Autodesk Inventor part; units mm, degrees
ref_plane "YZ Plane" through (0, 0, 0) normal (1, 0, 0) x (0, 1, 0)
ref_plane "XZ Plane" through (0, 0, 0) normal (0, 1, 0) x (-1, 0, 0)
ref_plane "XY Plane" through (0, 0, 0) normal (0, 0, 1) x (1, 0, 0)
sketch "Sketch1" plane through (0, 0, 0) normal (0, 1, 0) x (-1, 0, 0)
  line L0 (0, 0) -> (80, 0)
  line L1 (80, 0) -> (80, -40)
  line L2 (80, -40) -> (0, -40)
  line L3 (0, -40) -> (0, 0)
  line L4 (0, 0) -> (10, 0)
  line L5 (10, 0) -> (10, -10)
  line L6 (10, -10) -> (10, -30)
  circle A0 centre (10, -10) radius 3
  circle A1 centre (10, -30) radius 3
  line L7 (80, 0) -> (60, 0)
  line L8 (60, 0) -> (60, 30)
  line L9 (60, 30) -> (80, 30)
  line L10 (80, 30) -> (80, 0)
  dimension "d0" = 80
  dimension "d1" = 40
  dimension "d2" = 10
  dimension "d3" = 10
  dimension "d4" = 20
  dimension "d5" = 6
  dimension "d6" = 6
  dimension "d28" = 20
  dimension "d29" = 30
extrude "Extrusion1" add sketch "Sketch1" along normal blind 6
fillet "Fillet5" radius 5 6 edges at (-60, 3, 0) (-60, 3, 30) (-80, 3, 30) (0, 3, 0) (0, 3, -40) (-80, 3, -40)
fillet "Fillet6" radius 3 24 edges at (-1.4645, 6, -1.4645) (0, 6, -20) (-1.4645, 6, -38.5355) (-40, 6, -40) (-78.5355, 6, -38.5355) (-80, 6, -5) (-78.5355, 6, 28.5355) (-70, 6, 30) (-61.4645, 6, 28.5355) (-60, 6, 15) (-58.5355, 6, 1.4645) (-30, 6, 0) (-1.4645, 0, -1.4645) (0, 0, -20) (-1.4645, 0, -38.5355) (-40, 0, -40) (-78.5355, 0, -38.5355) (-80, 0, -5) (-78.5355, 0, 28.5355) (-70, 0, 30) (-61.4645, 0, 28.5355) (-60, 0, 15) (-58.5355, 0, 1.4645) (-30, 0, 0)
properties part number "CableHook"
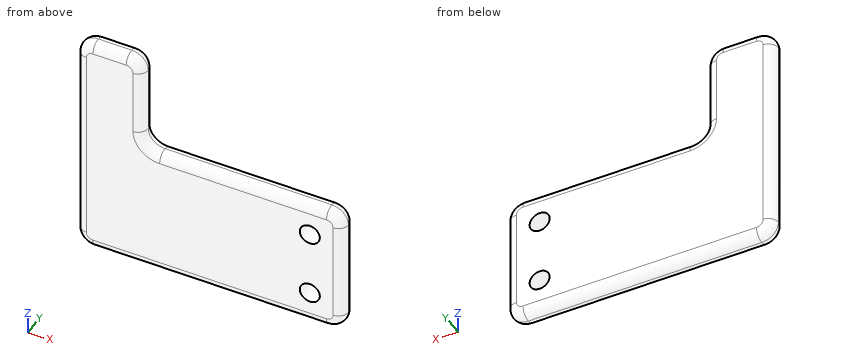
The listing builds one solid part. Answer for the finished solid, in the listing's coordinates (mm). Coordinates: 2 decimals unless noted, no trailing zeros.
Q1. Given P1, Ø9.5, axis at x = -10, z = -10, coming from the +Y side; P2, Ø1, axis at x = -22.5, y = 1.5, coming from the +Z side; P3, Ø2, axis at x = -27, y = 2, coming from the +Z side; P4, Ø1, axis at y = 2, z = 22.5, coming from the +X side, each flat-ended and moving along its own axis, determine where each tip first touches the part or whether it passes through.
Q2. A cutting plane is placed at B-B, the plane x = -10. State how many separate pieces and enclosed holes the cut face has, and give its area (3 significant figures).
Q3. Consider line 1 (Z direction, x = -10, y = 3.05); line 2 (X direction, y = 2.8, z = -10); line 3 (X direction, y = 3.85, z = -30). Determine where each line is inside the solid, lowest interval first.
Answers follow:
1. P1: stops at y = 6
1. P2: stops at z = -0.17
1. P3: stops at z = 0
1. P4: stops at x = -60.04
2. separate pieces: 3
2. enclosed holes: 0
2. area: 160 mm2
3. line 1: z = -40 to -33, -27 to -13, -7 to 0
3. line 2: x = -79.99 to -13, -7 to -0.01
3. line 3: x = -79.88 to -13, -7 to -0.12
